from build123d import *

# Parameters (mm, degrees)
SKETCH1_W                                  = 100
SKETCH1_H                                  = 70
BOSS_EXTRUDE1_DEPTH                        = 5
FILLET1_R                                  = 10
CUT_EXTRUDE1_REACH                         = 63.237
SKETCH2_R                                  = 1.85
MIRROR1_AT_THE_SECOND_PLANE_COPY_1_REACH   = 63.237
MIRROR1_AT_THE_SECOND_PLANE_COPY_1_SKETC_R = 1.85
CUT_EXTRUDE2_REACH                         = 63.237
SKETCH3_R                                  = 1.625
MIRROR2_AT_THE_SECOND_PLANE_COPY_1_REACH   = 63.237
MIRROR2_AT_THE_SECOND_PLANE_COPY_1_SKETC_R = 1.625
CUT_EXTRUDE3_REACH                         = 63.237
SKETCH4_W                                  = 70
SKETCH4_H                                  = 50
FILLET2_R                                  = 10
SKETCH5_R                                  = 3.125
CUT_EXTRUDE4_DEPTH                         = 3
MIRROR3_AT_THE_SECOND_PLANE_COPY_1_SKETC_R = 3.125
MIRROR3_AT_THE_SECOND_PLANE_COPY_1_DEPTH   = 3
SKETCH6_R                                  = 4
CUT_EXTRUDE5_DEPTH                         = 3
MIRROR4_AT_THE_SECOND_PLANE_COPY_1_SKETC_R = 4
MIRROR4_AT_THE_SECOND_PLANE_COPY_1_DEPTH   = 3
SKETCH9_W                                  = 15
SKETCH9_H                                  = 12.5
BOSS_EXTRUDE3_DEPTH                        = 20
CUT_EXTRUDE7_REACH                         = 109.819
SKETCH10_R                                 = 4
FILLET4_R                                  = 5


with BuildPart() as part:
    # Sketch1 → Boss-Extrude1 (new body)
    with BuildSketch(Plane(origin=(0, 0, 0), x_dir=(1, 0, 0), z_dir=(0, 1, 0))):
        Rectangle(SKETCH1_W, SKETCH1_H)
    extrude(amount=BOSS_EXTRUDE1_DEPTH)

    # Fillet1
    fillet1_edges = [part.edges().sort_by_distance(p)[0] for p in [
        (-50, 2.5, -35),
        (50, 2.5, -35),
        (50, 2.5, 35),
        (-50, 2.5, 35),
    ]]
    fillet(fillet1_edges, radius=FILLET1_R)

    # Sketch2 → Cut-Extrude1 (cut, up to next)
    with BuildSketch(Plane(origin=(0, 5, 0), x_dir=(1, 0, 0), z_dir=(0, 1, 0)), mode=Mode.PRIVATE) as cut_extrude1_sk1:
        with Locations(Location((-43, 13.5, 0), (0, 0, 270))):
            Circle(SKETCH2_R)
    cut_extrude1_tool1 = extrude(cut_extrude1_sk1.sketch, amount=-CUT_EXTRUDE1_REACH, mode=Mode.PRIVATE) & part.part
    cut_extrude1 = cut_extrude1_tool1.solids().sort_by_distance((-43, 5, -13.5))[0]
    add(cut_extrude1, mode=Mode.SUBTRACT)

    # Mirror1: Cut-Extrude1 across plane
    add(cut_extrude1.mirror(Plane(origin=(0, 0, 0), x_dir=(0, 0, 1), z_dir=(1, 0, 0))), mode=Mode.SUBTRACT)

    # Mirror1 at the second plane: Cut-Extrude1 across plane
    add(cut_extrude1.mirror(Plane.XY), mode=Mode.SUBTRACT)

    # Mirror1 at the second plane copy 1 sketc → Mirror1 at the second plane copy 1 (cut, up to next)
    with BuildSketch(Plane(origin=(0, 5, 0), x_dir=(-1, 0, 0), z_dir=(0, 1, 0)), mode=Mode.PRIVATE) as mirror1_at_the_second_plane_copy_1_sk1:
        with Locations(Location((-43, 13.5, 0), (0, 0, 270))):
            Circle(MIRROR1_AT_THE_SECOND_PLANE_COPY_1_SKETC_R)
    mirror1_at_the_second_plane_copy_1_tool1 = extrude(mirror1_at_the_second_plane_copy_1_sk1.sketch, amount=-MIRROR1_AT_THE_SECOND_PLANE_COPY_1_REACH, mode=Mode.PRIVATE) & part.part
    add(mirror1_at_the_second_plane_copy_1_tool1.solids().sort_by_distance((43, 5, 13.5))[0], mode=Mode.SUBTRACT)

    # Sketch3 → Cut-Extrude2 (cut, up to next)
    with BuildSketch(Plane(origin=(0, 5, 0), x_dir=(1, 0, 0), z_dir=(0, 1, 0)), mode=Mode.PRIVATE) as cut_extrude2_sk1:
        with Locations(Location((-24.5, 29, 0), (0, 0, 270))):
            Circle(SKETCH3_R)
    cut_extrude2_tool1 = extrude(cut_extrude2_sk1.sketch, amount=-CUT_EXTRUDE2_REACH, mode=Mode.PRIVATE) & part.part
    cut_extrude2 = cut_extrude2_tool1.solids().sort_by_distance((-24.5, 5, -29))[0]
    add(cut_extrude2, mode=Mode.SUBTRACT)

    # Mirror2: Cut-Extrude2 across plane
    add(cut_extrude2.mirror(Plane(origin=(0, 0, 0), x_dir=(0, 0, 1), z_dir=(1, 0, 0))), mode=Mode.SUBTRACT)

    # Mirror2 at the second plane: Cut-Extrude2 across plane
    add(cut_extrude2.mirror(Plane.XY), mode=Mode.SUBTRACT)

    # Mirror2 at the second plane copy 1 sketc → Mirror2 at the second plane copy 1 (cut, up to next)
    with BuildSketch(Plane(origin=(0, 5, 0), x_dir=(-1, 0, 0), z_dir=(0, 1, 0)), mode=Mode.PRIVATE) as mirror2_at_the_second_plane_copy_1_sk1:
        with Locations(Location((-24.5, 29, 0), (0, 0, 270))):
            Circle(MIRROR2_AT_THE_SECOND_PLANE_COPY_1_SKETC_R)
    mirror2_at_the_second_plane_copy_1_tool1 = extrude(mirror2_at_the_second_plane_copy_1_sk1.sketch, amount=-MIRROR2_AT_THE_SECOND_PLANE_COPY_1_REACH, mode=Mode.PRIVATE) & part.part
    add(mirror2_at_the_second_plane_copy_1_tool1.solids().sort_by_distance((24.5, 5, 29))[0], mode=Mode.SUBTRACT)

    # Sketch4 → Cut-Extrude3 (cut, up to next)
    with BuildSketch(Plane(origin=(0, 5, 0), x_dir=(1, 0, 0), z_dir=(0, 1, 0)), mode=Mode.PRIVATE) as cut_extrude3_sk1:
        Rectangle(SKETCH4_W, SKETCH4_H)
    cut_extrude3_tool1 = extrude(cut_extrude3_sk1.sketch, amount=-CUT_EXTRUDE3_REACH, mode=Mode.PRIVATE) & part.part
    add(cut_extrude3_tool1.solids().sort_by_distance((0, 5, 0))[0], mode=Mode.SUBTRACT)

    # Fillet2
    fillet2_edges = [part.edges().sort_by_distance(p)[0] for p in [
        (-35, 2.5, 25),
        (-35, 2.5, -25),
        (35, 2.5, -25),
        (35, 2.5, 25),
    ]]
    fillet(fillet2_edges, radius=FILLET2_R)

    # Sketch5 → Cut-Extrude4 (cut)
    with BuildSketch(Plane(origin=(0, 5, 0), x_dir=(1, 0, 0), z_dir=(0, 1, 0))):
        with Locations(Location((-24.5, 29, 0), (0, 0, 270))):
            Circle(SKETCH5_R)
    cut_extrude4 = extrude(amount=-CUT_EXTRUDE4_DEPTH, mode=Mode.SUBTRACT)

    # Mirror3: Cut-Extrude4 across plane
    add(cut_extrude4.mirror(Plane.XY), mode=Mode.SUBTRACT)

    # Mirror3 at the second plane: Cut-Extrude4 across plane
    add(cut_extrude4.mirror(Plane(origin=(0, 0, 0), x_dir=(0, 0, 1), z_dir=(1, 0, 0))), mode=Mode.SUBTRACT)

    # Mirror3 at the second plane copy 1 sketc → Mirror3 at the second plane copy 1 (cut)
    with BuildSketch(Plane(origin=(0, 5, 0), x_dir=(-1, 0, 0), z_dir=(0, 1, 0))):
        with Locations(Location((-24.5, 29, 0), (0, 0, 270))):
            Circle(MIRROR3_AT_THE_SECOND_PLANE_COPY_1_SKETC_R)
    extrude(amount=-MIRROR3_AT_THE_SECOND_PLANE_COPY_1_DEPTH, mode=Mode.SUBTRACT)

    # Sketch6 → Cut-Extrude5 (cut)
    with BuildSketch(Plane(origin=(0, 5, 0), x_dir=(1, 0, 0), z_dir=(0, 1, 0))):
        with Locations(Location((-43, 13.5, 0), (0, 0, 270))):
            Circle(SKETCH6_R)
    cut_extrude5 = extrude(amount=-CUT_EXTRUDE5_DEPTH, mode=Mode.SUBTRACT)

    # Mirror4: Cut-Extrude5 across plane
    add(cut_extrude5.mirror(Plane(origin=(0, 0, 0), x_dir=(0, 0, 1), z_dir=(1, 0, 0))), mode=Mode.SUBTRACT)

    # Mirror4 at the second plane: Cut-Extrude5 across plane
    add(cut_extrude5.mirror(Plane.XY), mode=Mode.SUBTRACT)

    # Mirror4 at the second plane copy 1 sketc → Mirror4 at the second plane copy 1 (cut)
    with BuildSketch(Plane(origin=(0, 5, 0), x_dir=(-1, 0, 0), z_dir=(0, 1, 0))):
        with Locations(Location((-43, 13.5, 0), (0, 0, 270))):
            Circle(MIRROR4_AT_THE_SECOND_PLANE_COPY_1_SKETC_R)
    extrude(amount=-MIRROR4_AT_THE_SECOND_PLANE_COPY_1_DEPTH, mode=Mode.SUBTRACT)

    # Sketch9 → Boss-Extrude3 (add)
    with BuildSketch(Plane.XZ):
        with Locations((-42.5, 0)):
            Rectangle(SKETCH9_W, SKETCH9_H)
        with Locations((42.5, 0)):
            Rectangle(SKETCH9_W, SKETCH9_H)
    extrude(amount=BOSS_EXTRUDE3_DEPTH)

    # Cut-Extrude7: up to this face of the body (flat: up to its plane)
    cut_extrude7_end = Plane(part.part.faces().sort_by_distance((50, -3.75, 0))[0])
    # Sketch10 → Cut-Extrude7 (cut, up to the picked face)
    with BuildSketch(Plane.ZY.offset(50), mode=Mode.PRIVATE) as cut_extrude7_sk1:
        with Locations((0, -12.5)):
            Circle(SKETCH10_R)
    cut_extrude7_tool1 = split(extrude(cut_extrude7_sk1.sketch, amount=-CUT_EXTRUDE7_REACH, mode=Mode.PRIVATE), bisect_by=cut_extrude7_end, keep=Keep.BOTH, mode=Mode.PRIVATE)
    add(cut_extrude7_tool1.solids().sort_by(Axis((-50, -12.5, 0), (1, 0, 0)))[0], mode=Mode.SUBTRACT)

    # Fillet4
    fillet4_edges = [part.edges().sort_by_distance(p)[0] for p in [
        (-42.5, 0, -6.25),
        (-42.5, 0, 6.25),
        (-42.5, -20, -6.25),
        (-42.5, -20, 6.25),
        (42.5, 0, -6.25),
        (42.5, 0, 6.25),
        (42.5, -20, -6.25),
        (42.5, -20, 6.25),
    ]]
    fillet(fillet4_edges, radius=FILLET4_R)


solid = part.part
Geometry: final body of the model. Coordinates: model frame, mm. A direction names the side the tool comes from. Give positions to 0.01 mm unless a question says otherwise; leave off trailing zeros. Write each loop counter-clockwise with the first axis right and the second up, starting at its lowest first coordinate (ties: lowest second). Pieces come first, ordered by that corner, then holes.
(1) Access query for faces 1 (the cylindrical face through (31.99, 2.46, 22.15)), 2 (the cylindrical face through (42.6, -1.43, 7.75)), 3 (the cylindrical face through (-47.15, 2.54, -31.99)), 4 (the flat face through (26, 2, 28)), 5 (the flat face through (42, -10, -6.25)). Directions: +Z, -Z, +X, -X, +Y, -Y. A direction counts if a zero-diameter tool reaches every point of the face in a straight line with its end or side. Return the directions, or none.
(2) First-contact query: P1, Ø3.5, axis at x = 24.5, z = 29, coming from the -Y side; P2, Ø5, axis at x = 39.5, y = -7.5, coming from the +Z side; P3, Ø8, axis at x = 44.5, y = -8.5, coming from the -Z side. Flat tips, straight axial feed; report the tip coordinate or a pass-through.
(3) Ray query, line 1 (Z direction, x = 24.5, y = 0.5) (3 decimals); line 2 (X direction, y = 0.75, z = -13.5); line 3 (Z direction, x = 24.5, y = 2.7) (3 decimals). Return the intervals inside material, ascending.
(4) Cut plane B-B, the plane z = -13.5. Return loops of the section in (x, y).
(5) Cut plane A-A, the plane x = -15. Return loops of the section in (y, z).
(6) Cut plane C-C, the plane y = -12.5. Return loops of the section in (x, z).
(7) Mould query, pull axis X, two halves, no side actions, for faces 6 (the flat face through (42, -20, 0)), 7 (the cylindrical face through (-44.641, 1.014, 12.646)), 8 (the flat face through (-50, -2, 0)). Classes: released by +X, released by -X, zero draft, split by the parting line, or undercut.
(8) Cut plane D-D, the plane x = 36.5. Return loops of the section in (y, z), then the cut area to 3 significant figures.
Values follow:
1. face 1: +Y, -Y
1. face 2: +Z, +X, -X, -Y
1. face 3: -Z, -X, +Y, -Y
1. face 4: +Y
1. face 5: -Z, +X, -X, -Y
2. P1: stops at y = 0
2. P2: stops at z = 6.25
2. P3: stops at z = -6.28
3. line 1: z = -35 to -30.625, -27.375 to -25, 25 to 27.375, 30.625 to 35
3. line 2: x = -50 to -44.85, -41.15 to -35, 35 to 41.15, 44.85 to 50
3. line 3: z = -35 to -32.125, -25.875 to -25, 25 to 25.875, 32.125 to 35
4. outline: (-50, 0) - (-44.85, 0) - (-44.85, 2) - (-47, 2) - (-47, 5) - (-50, 5) - close; (-41.15, 0) - (-35, 0) - (-35, 5) - (-39, 5) - (-39, 2) - (-41.15, 2) - close; (35, 0) - (41.15, 0) - (41.15, 2) - (39, 2) - (39, 5) - (35, 5) - close; (44.85, 0) - (50, 0) - (50, 5) - (47, 5) - (47, 2) - (44.85, 2) - close
5. outline: (0, -35) - (5, -35) - (5, -25) - (0, -25) - close; (0, 25) - (5, 25) - (5, 35) - (0, 35) - close
6. outline: (-50, -6.25) - (-35, -6.25) - (-35, -4) - (-50, -4) - close; (-50, 4) - (-35, 4) - (-35, 6.25) - (-50, 6.25) - close; (35, -6.25) - (50, -6.25) - (50, -4) - (35, -4) - close; (35, 4) - (50, 4) - (50, 6.25) - (35, 6.25) - close
7. face 6: zero draft
7. face 7: undercut
7. face 8: released by -X
8. outline: (-20, -1.25) arc R5 ccw to (-15, -6.25) - (-5, -6.25) arc R5 cw to (0, -11.25) - (0, -35) - (5, -35) - (5, 35) - (0, 35) - (0, 11.25) arc R5 cw to (-5, 6.25) - (-15, 6.25) arc R5 ccw to (-20, 1.25) - close; hole circle Ø8 at (-12.5, 0)
8. area: 550 mm2
